Check sheet for the modelled part. Datum: model origin and axes. Units: mm. Face numbers are marked on the shaded views. A direction names the side the tool comes from. Round coordinates to 2 decimals unless told otherwise and drop trailing zeros. Order: outer loops, then holes, each group sorted by start corner. A loop starts at its lowest first (then second) coordinate and runs counter-clockwise, first axis right, second up.
(1) Thickness scan on probe 1 along Y at (x, z) = (-7, -7.5); probe 2 along Y at (x, z) = (-11.5, -4.25); probe 3 along Z at (x, y) = (-0.25, 21). Record the ranges inside material, lowest first.
(2) Tool access check on the marked faces 1, 2 and 3. Record the directions out of +Z, -Z, +X, -X, +Y, -Y that give a thin tool (end or side, any length) a straight path to the whole face; none if there is none.
(3) Depth check by flat-ended pin: pin 1 (12 mm diameter, centred on x = 10, z = -2.5, fed in from +Y); pin 2 (10 mm diameter, centred on y = 83.5, z = -6, fed in from -X); pin 3 (3 mm diameter, centred on x = 6, y = 96, fed in from -Z). Enter the tip coordinate at first touch or a pass-through.
(4) Sectioned sample at C-C, the plane y = 59. Enter the section's corners in (x, z), and give its area (3 significant figures).
(5) Sectioned sample at D-D, the plane z = 5.5. Enter the section's corners in (x, y).
(6) Sectioned sample at A-A, the plane z = 0. Enter the section's corners in (x, y).
(7) Sectioned sample at B-B, the plane x = 0. Enter the section's corners in (y, z), and give its area (3 significant figures).
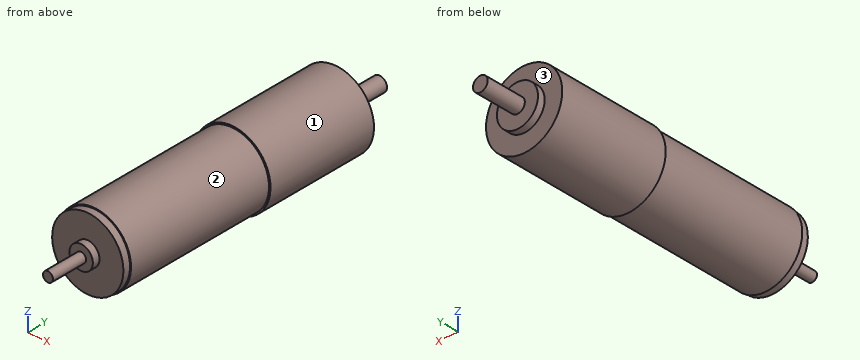
```python
from build123d import *

# Parameters (mm, degrees)
ESQUISSE2_R        = 1.692758077
BOSS_EXTRU_1_DEPTH = 15
ESQUISSE3_R        = 4
BOSS_EXTRU_2_DEPTH = 2.5


with BuildPart() as part:
    # Esquisse1 → Révolution1 (revolve)
    with BuildSketch(Plane.XY, mode=Mode.PRIVATE) as r_volution1_sk:
        Polygon((0, 0), (12.15, 0), (12.15, 2.5), (12.5, 2.5), (12.5, 54.5), (13, 54.5), (13, 93.5), (7, 93.5), (7, 96), (2.5, 96), (2.5, 110), (0, 110), align=None)
    revolve(r_volution1_sk.sketch.rotate(Axis((0, 0, 0), (0, 1, 0)), 90), axis=Axis((0, 0, 0), (0, 1, 0)))

    # Esquisse2 → Boss.-Extru.1 (add)
    with BuildSketch(Plane.XZ):
        with Locations(Location((0, 0, 0), (0, 0, 270))):
            Circle(ESQUISSE2_R)
    extrude(amount=BOSS_EXTRU_1_DEPTH)

    # Esquisse3 → Boss.-Extru.2 (add)
    with BuildSketch(Plane.XZ):
        with Locations(Location((0, 0, 0), (0, 0, 270))):
            Circle(ESQUISSE3_R)
    extrude(amount=BOSS_EXTRU_2_DEPTH)


solid = part.part
```
Derived:
1. probe 1: y = 0 to 93.5
1. probe 2: y = 2.5 to 93.5
1. probe 3: z = -12.5 to 12.5
2. face 1: +Y, -Y
2. face 2: -Y
2. face 3: +Y
3. pin 1: stops at y = 96
3. pin 2: stops at x = -12.96
3. pin 3: stops at z = -5.36
4. outline: circle Ø26 at (0, 0)
4. area: 531 mm2
5. outline: (-11.78, 54.5) - (-11.22, 54.5) - (-11.22, 2.5) - (-10.83, 2.5) - (-10.83, 0) - (10.83, 0) - (10.83, 2.5) - (11.22, 2.5) - (11.22, 54.5) - (11.78, 54.5) - (11.78, 93.5) - (4.33, 93.5) - (4.33, 96) - (-4.33, 96) - (-4.33, 93.5) - (-11.78, 93.5) - close
6. outline: (-13, 54.5) - (-12.5, 54.5) - (-12.5, 2.5) - (-12.15, 2.5) - (-12.15, 0) - (-4, 0) - (-4, -2.5) - (-1.69, -2.5) - (-1.69, -15) - (1.69, -15) - (1.69, -2.5) - (4, -2.5) - (4, 0) - (12.15, 0) - (12.15, 2.5) - (12.5, 2.5) - (12.5, 54.5) - (13, 54.5) - (13, 93.5) - (7, 93.5) - (7, 96) - (2.5, 96) - (2.5, 110) - (-2.5, 110) - (-2.5, 96) - (-7, 96) - (-7, 93.5) - (-13, 93.5) - close
7. outline: (-15, -1.69) - (-2.5, -1.69) - (-2.5, -4) - (0, -4) - (0, -12.15) - (2.5, -12.15) - (2.5, -12.5) - (54.5, -12.5) - (54.5, -13) - (93.5, -13) - (93.5, -7) - (96, -7) - (96, -2.5) - (110, -2.5) - (110, 2.5) - (96, 2.5) - (96, 7) - (93.5, 7) - (93.5, 13) - (54.5, 13) - (54.5, 12.5) - (2.5, 12.5) - (2.5, 12.15) - (0, 12.15) - (0, 4) - (-2.5, 4) - (-2.5, 1.69) - (-15, 1.69) - close
7. area: 2,540 mm2
